from build123d import *

# Parameters (mm, degrees)
CROQUIS1_W              = 5
CROQUIS1_H              = 2
SALIENTE_EXTRUIR1_DEPTH = 4
CROQUIS2_R              = 3
CORTAR_EXTRUIR1_DEPTH   = 6
SALIENTE_EXTRUIR2_START = 1.5
SALIENTE_EXTRUIR2_DEPTH = 1.5


with BuildPart() as part:
    # Croquis1 → Saliente-Extruir1 (new, symmetric)
    with BuildSketch(Plane.XY):
        with BuildLine():
            Line((5, 0), (8, 0))
            ThreePointArc((8, 0), (5.656854249, 5.656854249), (0, 8))
            Line((0, 8), (0, 0))
            Line((0, 0), (5, 0))
        make_face()
        with BuildLine():
            Line((0, 0), (0, 8))
            ThreePointArc((0, 8), (-5.656854249, 5.656854249), (-8, 0))
            Line((-8, 0), (-5, 0))
            Line((-5, 0), (0, 0))
        make_face()
        with BuildLine():
            Line((5, 0), (8, 0))
            ThreePointArc((8, 0), (5.656854249, 5.656854249), (0, 8))
            Line((0, 8), (0, 0))
            Line((0, 0), (5, 0))
        make_face()
        with BuildLine():
            Line((0, 0), (0, 8))
            ThreePointArc((0, 8), (-5.656854249, 5.656854249), (-8, 0))
            Line((-8, 0), (-5, 0))
            Line((-5, 0), (0, 0))
        make_face()
        with Locations((2.5, -1)):
            Rectangle(CROQUIS1_W, CROQUIS1_H)
        with Locations((-2.5, -1)):
            Rectangle(CROQUIS1_W, CROQUIS1_H)
    extrude(amount=SALIENTE_EXTRUIR1_DEPTH, both=True)

    # Croquis2 → Cortar-Extruir1 (cut)
    with BuildSketch(Plane.XZ.offset(2)):
        with Locations(Location((0, 0, 0), (0, 0, 270))):
            Circle(CROQUIS2_R)
    extrude(amount=-CORTAR_EXTRUIR1_DEPTH, mode=Mode.SUBTRACT)

    # Croquis3 → Saliente-Extruir2 (add)
    with BuildSketch(Plane.XY.offset(4).offset(SALIENTE_EXTRUIR2_START)):
        with BuildLine():
            Line((8, 0), (11, 0))
            ThreePointArc((11, 0), (0, 11), (-11, 0))
            Line((-11, 0), (-8, 0))
            ThreePointArc((-8, 0), (0, 8), (8, 0))
        make_face()
        with BuildLine():
            Line((-5, 0), (-5, -2))
            Line((-5, -2), (5, -2))
            Line((5, -2), (5, 0))
            Line((5, 0), (8, 0))
            ThreePointArc((8, 0), (0, 8), (-8, 0))
            Line((-8, 0), (-5, 0))
        make_face()
    saliente_extruir2 = extrude(amount=-SALIENTE_EXTRUIR2_DEPTH)

    # Simetría1: Saliente-Extruir2 across plane
    add(saliente_extruir2.mirror(Plane.XY))


solid = part.part
Geometry check sheet. Reference: the model listing, model coordinates, mm. A direction names the side the tool comes from. Round coordinates to 2 decimals unless told otherwise and drop trailing zeros. Order: outer loops, then holes, each group sorted by start corner. A loop starts at its lowest first (then second) coordinate and runs counter-clockwise, first axis right, second up. Notation, with made-up numbers: M 19.25,-20 L 24.25,-20 A9 cw 24.25,-15 Z; hole C 3.25,8 d2. An arc over 180 degrees is marked long. Answer in a Markdown table with one row per item.
(1) Go/stop test with flat-tipped pins: P1, Ø1.6, axis at y = -1.5, z = 0.5, coming from the -X side; P2, Ø3, axis at x = -1, z = 0, coming from the -Y side; P3, Ø1, axis at x = 5.5, z = 2, coming from the +Y side (3 decimals). Record where each tip stops, or that it passes through.
Responses:
| item | result |
|---|---|
| P1 | stops at x = -5 |
| P2 | stops at y = 4 |
| P3 | stops at y = 6.245 |
(2) Scan lines: probe 1 along X at (y, z) = (-0.7, 0); probe 2 along X at (y, z) = (0.05, 0); probe 3 along Z at (x, y) = (5, 7). Record each from-to range of solid material in increasing order. Write a range as from..to.
Responses:
| item | result |
|---|---|
| probe 1 | x = -5..-3, 3..5 |
| probe 2 | x = -8..-3, 3..8 |
| probe 3 | z = -5.5..-4, 4..5.5 |
(3) Sectioned sample at C-C, the plane y = 2. Record the cut outline in (x, z).
Responses:
| item | result |
|---|---|
| outline | M -10.82,-5.5 L 10.82,-5.5 L 10.82,-4 L 7.75,-4 L 7.75,4 L 10.82,4 L 10.82,5.5 L -10.82,5.5 L -10.82,4 L -7.75,4 L -7.75,-4 L -10.82,-4 Z; hole C 0,0 d6 |
(4) Sectioned sample at B-B, the plane x = 0. Record the cut outline in (y, z), and give its area (3 significant figures).
Responses:
| item | result |
|---|---|
| outline | M -2,-5.5 L 11,-5.5 L 11,-4 L 8,-4 L 8,4 L 11,4 L 11,5.5 L -2,5.5 L -2,3 L 4,3 L 4,-3 L -2,-3 Z |
| area | 83.0 mm² |
(5) Tool access check on faces 1 (the face through (-3, 8, 4)), 2 (the face through (-7, 0, 0)), 3 (the face through (7, 0, 0)). Record the directions out of +Z, -Z, +X, -X, +Y, -Y that give a thin tool (end or side, any length) a straight path to the whole face; none if there is none.
Responses:
| item | result |
|---|---|
| face 1 | +Y |
| face 2 | +Z, -Z, -X, -Y |
| face 3 | +Z, -Z, +X, -Y |
(6) Sectioned sample at A-A, the plane z = 0. Record the cut outline in (x, y).
Responses:
| item | result |
|---|---|
| outline | M -8,0 L -5,0 L -5,-2 L -3,-2 L -3,4 L 3,4 L 3,-2 L 5,-2 L 5,0 L 8,0 A8 ccw Z |
(7) Sectioned sample at D-D, the plane y = 4.25. Record the cut outline in (x, z), and give its area (3 significant figures).
Responses:
| item | result |
|---|---|
| outline | M -10.15,-5.5 L 10.15,-5.5 L 10.15,-4 L 6.78,-4 L 6.78,4 L 10.15,4 L 10.15,5.5 L -10.15,5.5 L -10.15,4 L -6.78,4 L -6.78,-4 L -10.15,-4 Z |
| area | 169 mm² |
(8) Draft check along Z on faces 4 (the face through (0, 5, 5.5)), 5 (the face through (0.9, 0.96, -2.86)), 6 (the face through (0, 11, 5)). Enter one of: released by +Z, released by -Z, zero draft, split by the parting line, or undercut.
Responses:
| item | result |
|---|---|
| face 4 | released by +Z |
| face 5 | undercut |
| face 6 | zero draft |
